from build123d import *

# Parameters (mm, degrees)
F1_DEPTH = 3


with BuildPart() as f1:
    # F0 (on Top) → F1 (new body)
    with BuildSketch(Plane.XY):
        Polygon((97.5, 26), (-17, 26), (-17, 16), (-20, 16), (-20, 3), (0, 3), (0, 0), (20, 0), (20, 3), (40, 3), (40, 0), (60, 0), (60, 3), (80, 3), (80, 0), (95, 0), (95, 3), (97.5, 3), align=None)
        with BuildLine():
            ThreePointArc((24.5, 6), (25.085786, 7.414214), (26.5, 8))
            Line((26.5, 8), (31.5, 8))
            ThreePointArc((31.5, 8), (32.914214, 7.414214), (33.5, 6))
            ThreePointArc((33.5, 6), (32.914214, 4.585786), (31.5, 4))
            Line((31.5, 4), (26.5, 4))
            ThreePointArc((26.5, 4), (25.085786, 4.585786), (24.5, 6))
        make_face(mode=Mode.SUBTRACT)
        Polygon((212, 26), (97.5, 26), (97.5, 3), (100, 3), (100, 0), (115, 0), (115, 3), (135, 3), (135, 0), (155, 0), (155, 3), (175, 3), (175, 0), (195, 0), (195, 3), (215, 3), (215, 16), (212, 16), align=None)
    extrude(amount=-F1_DEPTH)


solid = f1.part
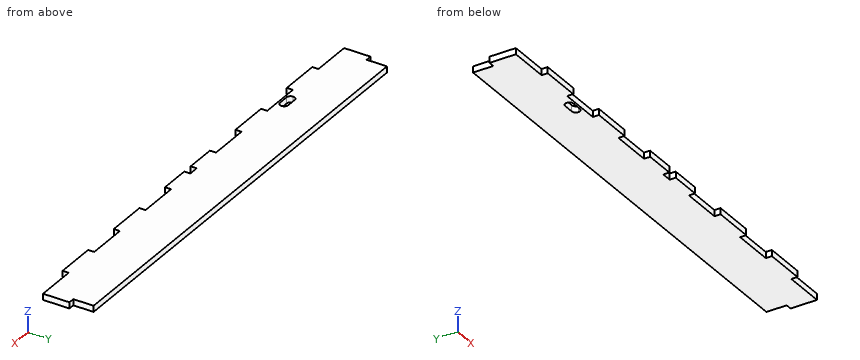
Geometry check sheet. Reference: the model listing, model coordinates, mm. Round coordinates to 2 decimals unless told otherwise and drop trailing zeros. Order: outer loops, then holes, each group sorted by start corner. A loop starts at its lowest first (then second) coordinate and runs counter-clockwise, first axis right, second up. Notation, with made-up numbers: (10.5, 45.25) - (44.5, 45.25) arc R24 ccw to (44.5, 60.25) - close; hole circle Ø2 at (82.25, 13.5). An arc over 180 degrees is marked (long way). One line per question, with ' | ' between items. Start each with the question number.
(1) Depth check by flat-ended pin: pin 1 Ø1.5 at (y, z) = (2, -2) entering from -X; pin 2 Ø0.9 at (x, z) = (-7, -2) entering from -Y; pin 3 Ø0.9 at (y, z) = (22, -2) entering from -X. Enter the tip coordinate at first touch or a pass-through.
(2) Sectioned sample at A-A on x = 68. Record the cut outline in (y, z).
(3) Sectioned sample at B-B on y = 20.75. Record the cut outline in (x, z), and give its area (3 significant figures).
(4) Thickness scan on L1, parallel to X at y = 2, z = -1.6; L2, parallel to X at y = 20.25, z = -2.5; L3, parallel to Y at x = 131, z = -0.9. Record the ranges inside material, lowest first. Write a range as [from, to].
Conclusion:
1) pin 1: stops at x = 0 | pin 2: stops at y = 3 | pin 3: stops at x = -17
2) outline: (3, -3) - (26, -3) - (26, 0) - (3, 0) - close
3) outline: (-17, -3) - (212, -3) - (212, 0) - (-17, 0) - close | area: 687 mm2
4) L1: x = [0, 20], [40, 60], [80, 95], [100, 115], [135, 155], [175, 195] | L2: x = [-17, 212] | L3: y = [3, 26]
